Check sheet for the modelled part. Datum: model origin and axes. Units: mm. Face numbers are marked on the shaded views. A direction names the side the tool comes from. Give positions to 0.01 mm unless a question says otherwise; leave off trailing zeros. Write each loop counter-clockwise with the first axis right and the second up, starting at its lowest first coordinate (ties: lowest second). Pieces come first, ordered by that corner, then holes. Notation, with made-up numbers: M -7,-30 L 26,-30 A26 ccw 26,6 Z; hole C -37,51 d6. An arc over 180 degrees is marked long. Write item = value, one per line. Start each with the question number.
1) Cross-section at B-B, the plane x = 15. Record the cut outline in (y, z), plus the area to 3 significant figures.
2) Cross-section at D-D, the plane x = 0. Record the cut outline in (y, z).
3) Go/stop test with flat-tipped pins: pin 1 (1 mm diameter, centred on x = 7.5, y = 7, fed in from -Z); pin 2 (1.5 mm diameter, centred on x = -2.5, y = 2, fed in from -Z); pin 3 (2.5 mm diameter, centred on x = 14.295, z = 0, fed in from -Y); pin 4 (4 mm diameter, centred on x = -13.5, y = 4, fed in from -Z). Record where each tip stops, or that it passes through.
4) Mould release check, pull along X, two halves, no side actions. Record for the marked faces 1, 2 and 3: released by +X, released by -X, zero draft, split by the parting line, or undercut.
5) Scan lines: line 1 along X through (y, z) = (5.75, 0) (3 decimals); line 2 along X through (y, z) = (0.75, -1); line 3 along Z through (x, y) = (15.5, 2.5). Record each from-to range of solid material in increasing order. Write a range as [from, to].
6) Cross-section at C-C, the plane y = 6.25. Give the number of separate pieces and of enclosed holes in the cut face, plus the area to 3 significant figures.
7) Cross-section at A-A, the plane z = 0. Record the cut outline in (x, y) (3 decimals).
8) Access from +Z, -Z, +X, -X, +Y, -Y to the whole of each face (thin tool, end or side, straight path). Record for the marked faces 4, 5, 6 and 7.
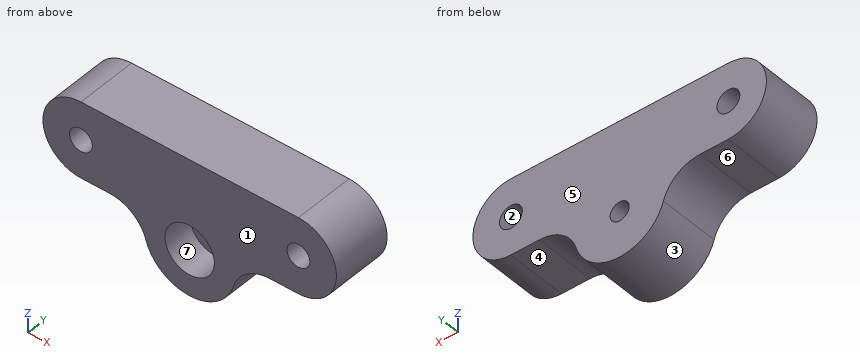
```python
from build123d import *

# Parameters (mm, degrees)
SKETCH_1_R          = 1.5
EXTRUDE_1_DEPTH     = 8
EXTRUDE_2_DEPTH     = 8
SKETCH_3_R          = 3.25
CUT_EXTRUDE_1_DEPTH = 4
FILLET_1_R          = 5
HOLE_WIZARD_M3_1_D  = 2.5


with BuildPart() as part:
    # 草图1 → 凸台-拉伸1 (new body)
    with BuildSketch(Plane(origin=(0, 0, 0), x_dir=(1, 0, 0), z_dir=(0, 1, 0))):
        with BuildLine():
            Line((-14.295, 5), (14.295, 5))
            ThreePointArc((14.295, 5), (19.295, 0), (14.295, -5))
            Line((14.295, -5), (-14.295, -5))
            ThreePointArc((-14.295, -5), (-19.295, 0), (-14.295, 5))
        make_face()
        with Locations(Location((-14.295, 0, 0), (0, 0, 270))):
            Circle(SKETCH_1_R, mode=Mode.SUBTRACT)
        with Locations(Location((14.295, 0, 0), (0, 0, 270))):
            Circle(SKETCH_1_R, mode=Mode.SUBTRACT)
    extrude(amount=EXTRUDE_1_DEPTH)

    # 草图2 → 凸台-拉伸2 (add)
    with BuildSketch(Plane(origin=(0, 8, 0), x_dir=(1, 0, 0), z_dir=(0, 1, 0))):
        with BuildLine():
            Line((-6, 6.88), (-6, 5))
            Line((-6, 5), (6, 5))
            Line((6, 5), (6, 6.88))
            ThreePointArc((6, 6.88), (0, 12.88), (-6, 6.88))
        make_face()
    extrude(amount=-EXTRUDE_2_DEPTH)

    # 草图3 → 切除-拉伸1 (cut)
    with BuildSketch(Plane.XZ):
        with Locations(Location((0, -6.88, 0), (0, 0, 270))):
            Circle(SKETCH_3_R)
    extrude(amount=-CUT_EXTRUDE_1_DEPTH, mode=Mode.SUBTRACT)

    # 圆角1
    fillet_1_edges = [part.edges().sort_by_distance(p)[0] for p in [
        (-6, 4, -5),
        (6, 4, -5),
    ]]
    fillet(fillet_1_edges, radius=FILLET_1_R)

    # M3 螺纹孔1 (through all)
    with Locations(Plane(origin=(0, 4, -6.88), x_dir=(0, 0, -1), z_dir=(0, -1, 0))):
        with Locations((0, 0)):
            Hole(HOLE_WIZARD_M3_1_D / 2)


solid = part.part
```
Reply:
q1.outline = M 0,-4.95 L 8,-4.95 L 8,-1.32 L 0,-1.32 Z; M 0,1.32 L 8,1.32 L 8,4.95 L 0,4.95 Z
q1.area = 58.0 mm2
q2.outline = M 0,-12.88 L 8,-12.88 L 8,-8.13 L 4,-8.13 L 4,-10.13 L 0,-10.13 Z; M 0,-3.63 L 4,-3.63 L 4,-5.63 L 8,-5.63 L 8,5 L 0,5 Z
q3.pin_1 = -6.48
q3.pin_2 = -12.62
q3.pin_3 = through
q3.pin_4 = -5
q4.face_1 = zero draft
q4.face_2 = undercut
q4.face_3 = split by the parting line
q5.line_1 = [-19.295, -15.795], [-12.795, 12.795], [15.795, 19.295]
q5.line_2 = [-19.19, -15.41], [-13.18, 13.18], [15.41, 19.19]
q5.line_3 = [-4.85, -0.89], [0.89, 4.85]
q6.separate_pieces = 1
q6.enclosed_holes = 3
q6.area = 432 mm2
q7.outline = M -19.295,0 L -15.795,0 L -15.795,8 L -19.295,8 Z; M -12.795,0 L 12.795,0 L 12.795,8 L -12.795,8 Z; M 15.795,0 L 19.295,0 L 19.295,8 L 15.795,8 Z
q8.face_4 = -Z, +X, +Y, -Y
q8.face_5 = +Z, -Z, +X, -X, +Y
q8.face_6 = -Z, -X, +Y, -Y
q8.face_7 = -Y
